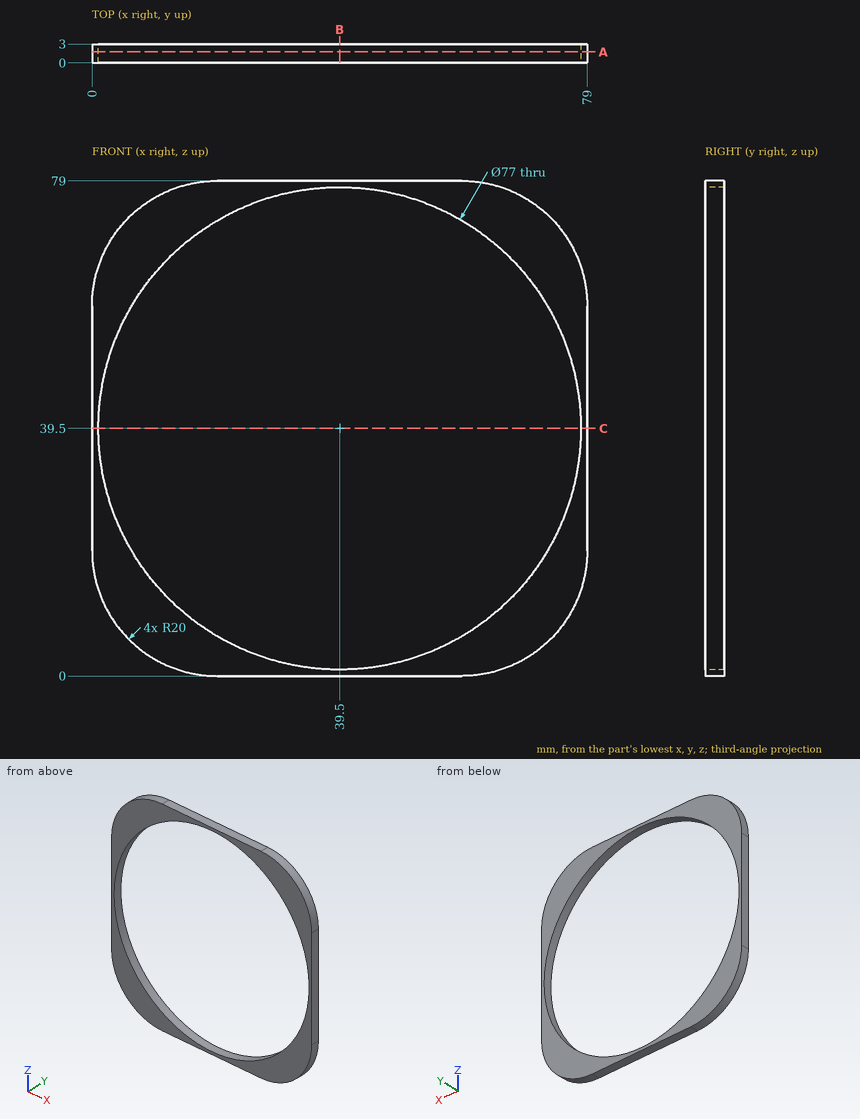
Geometry check sheet. Reference: drawing and pictorial views, mm from the part's lowest x, y, z. Give positions to 0.01 mm unless a question says otherwise; leave off trailing zeros. Write each loop counter-clockwise with the first axis right and the second up, starting at its lowest first coordinate (ties: lowest second). Pieces come first, ordered by that corner, then holes. Notation, with made-up numbers: M -13,67 L -4,67 A12 ccw -4,84 Z; hole C -20,54 d3. An arc over 180 degrees is marked long. Put each result on its own line as item: value. Start each with the question number.
1. Scan lines: line 1 along Z through (x, y) = (39.5, 2.3); line 2 along Z through (x, y) = (56, 1.25); line 3 along X through (y, z) = (2.5, 47). Record each from-to range of solid material in increasing order. Write a range as [from, to].
2. Section check A-A (y = 1.75). Record the cut outline in (x, z).
3. Section check B-B (x = 39.5). Record the cut outline in (y, z).
4. Section check C-C (z = 39.5). Record the cut outline in (x, y).
5. Go/stop test with a flat-tipped pin: pin 1 Ø1.5 at (y, z) = (1, 60.5) entering from -X. Record where the tip stops, or that it passes through.
Answer list:
1. line 1: [0, 1], [78, 79]
1. line 2: [0, 4.71], [74.29, 79]
1. line 3: [0, 1.74], [77.26, 79]
2. outline: M 0,20 A20 ccw 20,0 L 59,0 A20 ccw 79,20 L 79,59 A20 ccw 59,79 L 20,79 A20 ccw 0,59 Z; hole C 39.5,39.5 d77
3. outline: M 0,0 L 3,0 L 3,1 L 0,1 Z; M 0,78 L 3,78 L 3,79 L 0,79 Z
4. outline: M 0,0 L 1,0 L 1,3 L 0,3 Z; M 78,0 L 79,0 L 79,3 L 78,3 Z
5. pin 1: x = 0.01
